Work out the finished part from the listing and answer in its coordinate system (mm). Face numbers are marked on the shaded views. A direction names the side the tool comes from. Round coordinates to 2 decimals unless told otherwise and drop trailing zeros. Write each loop counter-clockwise with the first axis right and the second up, starting at its lowest first coordinate (ties: lowest second). Pieces come first, ordered by that corner, then holes. Notation, with made-up numbers: M 86.25,-33 L 137.25,-33 A15 ccw 137.25,-8 Z; hole C 5.5,71.5 d4. An arc over 180 degrees is marked long. Answer in a Markdown table with one row per item.
```python
from build123d import *

# Parameters (mm, degrees)
BOSS_EXTRUDE1_OUTLINE_R   = 1.426531271
BOSS_EXTRUDE1_OUTLINE_R_2 = 1.343679746
BOSS_EXTRUDE1_OUTLINE_R_3 = 1.378285228
BOSS_EXTRUDE1_OUTLINE_R_4 = 1.385856135
BOSS_EXTRUDE1_DEPTH       = 2.5
BOSS_EXTRUDE2_START       = -3
SKETCH1_3_R               = 3
SKETCH1_3_R_2             = 1.378285228
SKETCH1_3_R_3             = 1.385856135
SKETCH1_3_R_4             = 1.343679746
SKETCH1_3_R_5             = 1.426531271
BOSS_EXTRUDE2_DEPTH       = 3
FILLET1_R                 = 3


# Read off the part's stored shape, not the designer's step: Boss-Extrude1
with BuildPart() as part:
    # Boss-Extrude1 outline → Boss-Extrude1 (new body)
    with BuildSketch(Plane(origin=(0, 0, 0), x_dir=(1, 0, 0), z_dir=(0, 1, 0))):
        with BuildLine():
            Line((-76.498848721, -45), (76.503120692, -45.002303107))
            ThreePointArc((76.503120692, -45.002303107), (78.976602231, -43.977753507), (80.001151831, -41.504271968))
            Line((80.001151831, -41.504271968), (80.001151831, 41.501969416))
            ThreePointArc((80.001151831, 41.501969416), (78.977276633, 43.973822805), (76.505423244, 44.997698002))
            Line((76.505423244, 44.997698002), (-76.373794917, 44.999998119))
            ThreePointArc((-76.373794917, 44.999998119), (-78.930513463, 44.02078083), (-79.998848724, 41.5))
            Line((-79.998848724, 41.5), (-80.001153885, -41.501969416))
            ThreePointArc((-80.001153885, -41.501969416), (-78.975092852, -43.976962316), (-76.498848721, -45))
        make_face()
        with Locations((-52.498848724, -37)):
            Circle(BOSS_EXTRUDE1_OUTLINE_R, mode=Mode.SUBTRACT)
        with Locations((69.001151276, -37)):
            Circle(BOSS_EXTRUDE1_OUTLINE_R_2, mode=Mode.SUBTRACT)
        with Locations((-52.498848724, 32)):
            Circle(BOSS_EXTRUDE1_OUTLINE_R_3, mode=Mode.SUBTRACT)
        with Locations((69.001151276, 32)):
            Circle(BOSS_EXTRUDE1_OUTLINE_R_4, mode=Mode.SUBTRACT)
    extrude(amount=BOSS_EXTRUDE1_DEPTH)

    # Sketch1<3> → Boss-Extrude2 (add)
    # profile 1 of 4: a face of its own
    with BuildSketch(Plane(origin=(0, 0, 0), x_dir=(1, 0, 0), z_dir=(0, 1, 0)).offset(BOSS_EXTRUDE2_START)):
        with Locations(Location((-52.498848724, 32, 0), (0, 0, 270))):
            Circle(SKETCH1_3_R)
        with Locations(Location((-52.498848724, 32, 0), (0, 0, 270))):
            Circle(SKETCH1_3_R_2, mode=Mode.SUBTRACT)
    # profile 2 of 4: a face of its own
    with BuildSketch(Plane(origin=(0, 0, 0), x_dir=(1, 0, 0), z_dir=(0, 1, 0)).offset(BOSS_EXTRUDE2_START)):
        with Locations(Location((69.001151276, 32, 0), (0, 0, 270))):
            Circle(SKETCH1_3_R)
        with Locations(Location((69.001151276, 32, 0), (0, 0, 270))):
            Circle(SKETCH1_3_R_3, mode=Mode.SUBTRACT)
    # profile 3 of 4: a face of its own
    with BuildSketch(Plane(origin=(0, 0, 0), x_dir=(1, 0, 0), z_dir=(0, 1, 0)).offset(BOSS_EXTRUDE2_START)):
        with Locations(Location((69.001151276, -37, 0), (0, 0, 270))):
            Circle(SKETCH1_3_R)
        with Locations(Location((69.001151276, -37, 0), (0, 0, 270))):
            Circle(SKETCH1_3_R_4, mode=Mode.SUBTRACT)
    # profile 4 of 4: a face of its own
    with BuildSketch(Plane(origin=(0, 0, 0), x_dir=(1, 0, 0), z_dir=(0, 1, 0)).offset(BOSS_EXTRUDE2_START)):
        with Locations(Location((-52.498848724, -37, 0), (0, 0, 270))):
            Circle(SKETCH1_3_R)
        with Locations(Location((-52.498848724, -37, 0), (0, 0, 270))):
            Circle(SKETCH1_3_R_5, mode=Mode.SUBTRACT)
    extrude(amount=BOSS_EXTRUDE2_DEPTH)

    # Fillet1
    fillet1_edges = [part.edges().sort_by_distance(p)[0] for p in [
        (-52.498848724, 0, -35),
        (69.001151276, 0, -35),
        (69.001151276, 0, 34),
        (-52.498848724, 0, 34),
    ]]
    fillet(fillet1_edges, radius=FILLET1_R - 0.0001)  # a hair under: the kernel refuses the full size


solid = part.part
```
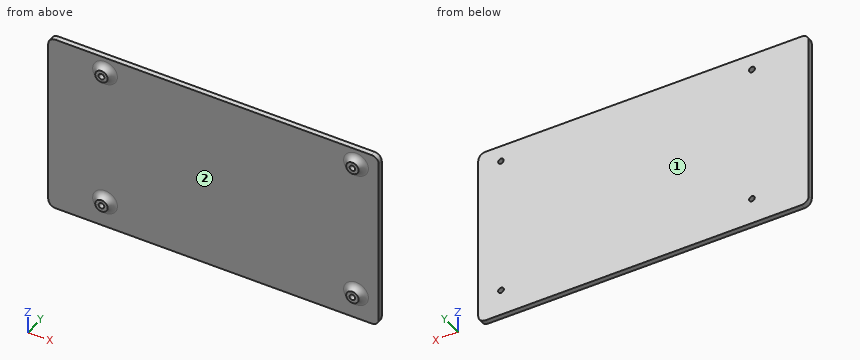
1. The part is cut by section C-C (x = -4.5). Determine the outline of the cut face in (y, z), plus the area to 3 significant figures.
Calculated:
| item | result |
|---|---|
| outline | M 0,-45 L 2.5,-45 L 2.5,45 L 0,45 Z |
| area | 225 mm² |
2. Consider line 1 along X through (y, z) = (0.4, -32); line 2 along X through (y, z) = (0.1, 37); line 3 along X through (y, z) = (-1.45, -32). Determine where each line is inside the solid, lowest interval first. Write a range as from..to.
Calculated:
| item | result |
|---|---|
| line 1 | x = -80..-53.88, -51.12..67.62, 70.39..80 |
| line 2 | x = -80..-53.93, -51.07..67.66, 70.34..80 |
| line 3 | x = -55.93..-53.88, -51.12..-49.07, 65.57..67.62, 70.39..72.43 |
3. The part is cut by section A-A (y = -1.1). Determine the outline of the cut face in (x, z), plus the area to 3 significant figures.
Calculated:
| item | result |
|---|---|
| outline | C -52.5,-32 d7.36; C -52.5,37 d7.36; C 69,-32 d7.36; C 69,37 d7.36; hole C -52.5,37 d2.85; hole C -52.5,-32 d2.76; hole C 69,-32 d2.77; hole C 69,37 d2.69 |
| area | 146 mm² |
4. Given pin 1 (2 mm diameter, centred on x = 10, y = 2, fed in from -Z); pin 2 (6 mm diameter, centred on x = 38.5, z = -26, fed in from -Y), each flat-ended and moving along its own axis, determine where each tip first touches the part or whether it passes through.
Calculated:
| item | result |
|---|---|
| pin 1 | stops at z = -45 |
| pin 2 | stops at y = 0 |
5. A tool of negligible diameter and unlimited length cuts with its end or side. For the marked faces 1 and 2, from which of +Z, -Z, +X, -X, +Y, -Y can it reach the whole face along a straight path? Write none if from no direction.
Calculated:
| item | result |
|---|---|
| face 1 | +Z, -Z, +X, -X, +Y |
| face 2 | -Y |
6. The part is cut by section B-B (z = 11). Determine the outline of the cut face in (x, y), plus the area to 3 significant figures.
Calculated:
| item | result |
|---|---|
| outline | M -80,0 L 80,0 L 80,2.5 L -80,2.5 Z |
| area | 400 mm² |
